```python
from build123d import *

# Parameters (mm, degrees)
SKETCH1_W           = 18.1
SKETCH1_H           = 18.4
BOSS_EXTRUDE1_DEPTH = 0.4
SKETCH2_W           = 18
SKETCH2_H           = 18
BOSS_EXTRUDE2_DEPTH = 2.2
SKETCH3_W           = 6.15
SKETCH3_H           = 4.3
BOSS_EXTRUDE3_DEPTH = 3
SKETCH4_W           = 5.15
SKETCH4_H           = 2
CUT_EXTRUDE1_DEPTH  = 3.5
SKETCH5_W           = 17.2
SKETCH5_H           = 11.5
BOSS_EXTRUDE4_DEPTH = 2.2
FILLET1_R           = 0.25
SKETCH6_R           = 2.35
BOSS_EXTRUDE5_DEPTH = 1.7
FILLET2_R           = 0.5
CHAMFER1_SIZE       = 0.25
FILLET3_R           = 0.5


with BuildPart() as part:
    # Sketch1 → Boss-Extrude1 (new body, symmetric)
    with BuildSketch(Plane(origin=(0, 0, 0), x_dir=(1, 0, 0), z_dir=(0, 1, 0))):
        Rectangle(SKETCH1_W, SKETCH1_H)
    extrude(amount=BOSS_EXTRUDE1_DEPTH, both=True)

    # Sketch2 → Boss-Extrude2 (add)
    with BuildSketch(Plane(origin=(0, 0.4, 0), x_dir=(1, 0, 0), z_dir=(0, 1, 0))):
        Rectangle(SKETCH2_W, SKETCH2_H)
    extrude(amount=BOSS_EXTRUDE2_DEPTH)

    # Sketch3 → Boss-Extrude3 (add)
    with BuildSketch(Plane.XZ.offset(0.4)):
        with Locations((0, -6.55)):
            Rectangle(SKETCH3_W, SKETCH3_H)
    extrude(amount=BOSS_EXTRUDE3_DEPTH)

    # Sketch4 → Cut-Extrude1 (cut)
    with BuildSketch(Plane(origin=(0, 0, -8.7), x_dir=(-1, 0, 0), z_dir=(0, 0, -1))):
        with Locations((0, -1.9)):
            Rectangle(SKETCH4_W, SKETCH4_H)
    extrude(amount=-CUT_EXTRUDE1_DEPTH, mode=Mode.SUBTRACT)

    # Sketch5 → Boss-Extrude4 (add)
    with BuildSketch(Plane.XZ.offset(0.4)):
        with Locations((0, 2.95)):
            Rectangle(SKETCH5_W, SKETCH5_H)
    extrude(amount=BOSS_EXTRUDE4_DEPTH)

    # Fillet1
    fillet1_edges = [part.edges().sort_by_distance(p)[0] for p in [
        (8.6, -2.6, 2.95),
        (0, -2.6, 8.7),
        (-8.6, -2.6, 2.95),
        (0, -2.6, -2.8),
    ]]
    fillet(fillet1_edges, radius=FILLET1_R)

    # Sketch6 → Boss-Extrude5 (add)
    with BuildSketch(Plane.XZ.offset(0.4)):
        with Locations((6.5, -6.65)):
            Circle(SKETCH6_R)
    extrude(amount=BOSS_EXTRUDE5_DEPTH)

    # Fillet2
    fillet2_edges = [part.edges().sort_by_distance(p)[0] for p in [
        (-9, 1.5, -9),
        (-9, 1.5, 9),
        (9, 1.5, 9),
        (9, 1.5, -9),
    ]]
    fillet(fillet2_edges, radius=FILLET2_R)

    # Chamfer1
    chamfer1_edges = [part.edges().sort_by_distance(p)[0] for p in [
        (-9, 2.6, 0),
        (0, 2.6, -9),
        (0, 2.6, 9),
        (9, 2.6, 0),
        (8.853553391, 2.6, -8.853553391),
        (8.853553391, 2.6, 8.853553391),
        (-8.853553391, 2.6, 8.853553391),
        (-8.853553391, 2.6, -8.853553391),
    ]]
    chamfer(chamfer1_edges, length=CHAMFER1_SIZE)

    # Fillet3
    fillet3_edges = [part.edges().sort_by_distance(p)[0] for p in [
        (-9.05, 0, -9.2),
        (9.05, 0, -9.2),
    ]]
    fillet(fillet3_edges, radius=FILLET3_R)


solid = part.part
```
Geometry check sheet. Reference: the model listing, model coordinates, mm. A direction names the side the tool comes from. Round coordinates to 2 decimals unless told otherwise and drop trailing zeros. Order: outer loops, then holes, each group sorted by start corner. A loop starts at its lowest first (then second) coordinate and runs counter-clockwise, first axis right, second up. Notation, with made-up numbers: M 24,40.25 L 75,40.25 A16 cw 75,54.25 Z; hole C 52,-25 d6. An arc over 180 degrees is marked long. Answer as CSV lines item,"result".
1) Sectioned sample at C-C on x = 0.25. Record the cut outline in (y, z).
Entries:
outline,"M -3.4,-8.7 L -2.9,-8.7 L -2.9,-5.2 L -0.9,-5.2 L -0.9,-8.7 L -0.4,-8.7 L -0.4,-9.2 L 0.4,-9.2 L 0.4,-9 L 2.35,-9 L 2.6,-8.75 L 2.6,8.75 L 2.35,9 L 0.4,9 L 0.4,9.2 L -0.4,9.2 L -0.4,8.7 L -2.35,8.7 A0.25 ccw -2.6,8.45 L -2.6,-2.55 A0.25 ccw -2.35,-2.8 L -0.4,-2.8 L -0.4,-4.4 L -3.4,-4.4 Z"
2) Sectioned sample at B-B on z = -6.65. Record the cut outline in (x, y) (3 decimals).
Entries:
outline,"M -9.05,-0.4 L -3.075,-0.4 L -3.075,-3.4 L 3.075,-3.4 L 3.075,-0.4 L 4.15,-0.4 L 4.15,-2.1 L 8.85,-2.1 L 8.85,-0.4 L 9.05,-0.4 L 9.05,0.4 L 9,0.4 L 9,2.35 L 8.75,2.6 L -8.75,2.6 L -9,2.35 L -9,0.4 L -9.05,0.4 Z; hole M -2.575,-2.9 L 2.575,-2.9 L 2.575,-0.9 L -2.575,-0.9 Z"
3) Sectioned sample at A-A on y = -1.15. Record the cut outline in (x, z) (3 decimals).
Entries:
outline,"M -8.6,-2.8 L 8.6,-2.8 L 8.6,8.7 L -8.6,8.7 Z; M -3.075,-8.7 L -2.575,-8.7 L -2.575,-5.2 L 2.575,-5.2 L 2.575,-8.7 L 3.075,-8.7 L 3.075,-4.4 L -3.075,-4.4 Z; C 6.5,-6.65 d4.7"
4) Gauge pin test, flat ends, axial feed: pin 1 Ø0.6 at (y, z) = (1, -1.5) entering from -X; pin 2 Ø1.6 at (y, z) = (-1.5, 1) entering from -X; pin 3 Ø1.5 at (x, y) = (0.5, -1.5) entering from +Z. Record the tip position at first contact, or that the pin passes through.
Entries:
pin 1,"x = -9"
pin 2,"x = -8.6"
pin 3,"z = 8.7"
5) Tool access check on faces 4 (the face through (8.6, -1, 3)), 5 (the face through (0, -2.6, 3)), 6 (the face through (0, -0.9, -7)). Record the directions out of +Z, -Z, +X, -X, +Y, -Y that give a thin tool (end or side, any length) a straight path to the whole face; none if there is none.
Entries:
face 4,"+Z, +X, -Y"
face 5,"+Z, +X, -X, -Y"
face 6,"-Z"
6) Thickness scan on probe 1 along X at (y, z) = (-0.95, -6.5) (3 decimals); probe 2 along Y at (x, z) = (0.75, -6); probe 3 along Y at (x, z) = (7.75, -6.5). Record the ranges inside material, lowest first. Write a range as [from, to].
Entries:
probe 1,"[-3.075, -2.575], [2.575, 3.075], [4.155, 8.845]"
probe 2,"[-3.4, -2.9], [-0.9, 2.6]"
probe 3,"[-2.1, 2.6]"
7) Mould release check, pull along X, two halves, no side actions. Record for faces 1 (the face through (0, 1, -9)), 2 (the face through (-9, 1, 0)), 3 (the face through (3.075, -2, -7)): +X half, -X half, draft (parallel to the pull), parting line (faces both ways), or undercut.
Entries:
face 1,"draft"
face 2,"-X half"
face 3,"undercut"
8) Sectioned sample at D-D on y = 1.3. Record the cut outline in (x, z), and give its area (3 significant figures).
Entries:
outline,"M -9,-8.5 A0.5 ccw -8.5,-9 L 8.5,-9 A0.5 ccw 9,-8.5 L 9,8.5 A0.5 ccw 8.5,9 L -8.5,9 A0.5 ccw -9,8.5 Z"
area,"324 mm2"
